For this review, use the dimensioned drawing (mm, ordinates from the lowest corner) and the shaded views. A direction names the side the tool comes from. Give positions to 0.01 mm unless a question says otherwise; leave off trailing zeros. Loops run counter-clockwise (first coordinate to the right, second up) from the corner with the lowest first, then second, coordinate; pieces in that order, holes last. Notation, with made-up numbers: M -16,-29 L 34,-29 A26 ccw 34,5 Z; hole C 65,-13.75 d1. An arc over 180 degrees is marked long. Use a Markdown table: item, result. Add a question column.
(1) For probe 1 along Z at (x, y) = (39, 13); probe 2 along Y at (x, z) = (55.5, 9.5) (1 decimal); probe 3 along Z at (x, y) = (60, 71.5) (1 decimal), list the stretches that pass through material, from the lowest coordinate up.
(2) Add section A-A, the plane z = 27. Give the boundary of the cut face in (x, y).
(3) For the marked faces 1 and 2, list the 3-axis set-ups (+Z, -Z, +X, -X, +Y, -Y) from which the entire face can be reached by the end or side of a thin tool; tool diameter is ignored.
(4) Insertion check: pin 1 Ø10 at (y, z) = (51, 18.5) entering from -X (1 decimal); pin 2 Ø10 at (y, z) = (25, 19) entering from -X (1 decimal); pin 3 Ø6 at (y, z) = (44, 33) entering from -X. Each pin has a flat end and moves straight along its axis. Give the tip position at first contact, or say it passes through.
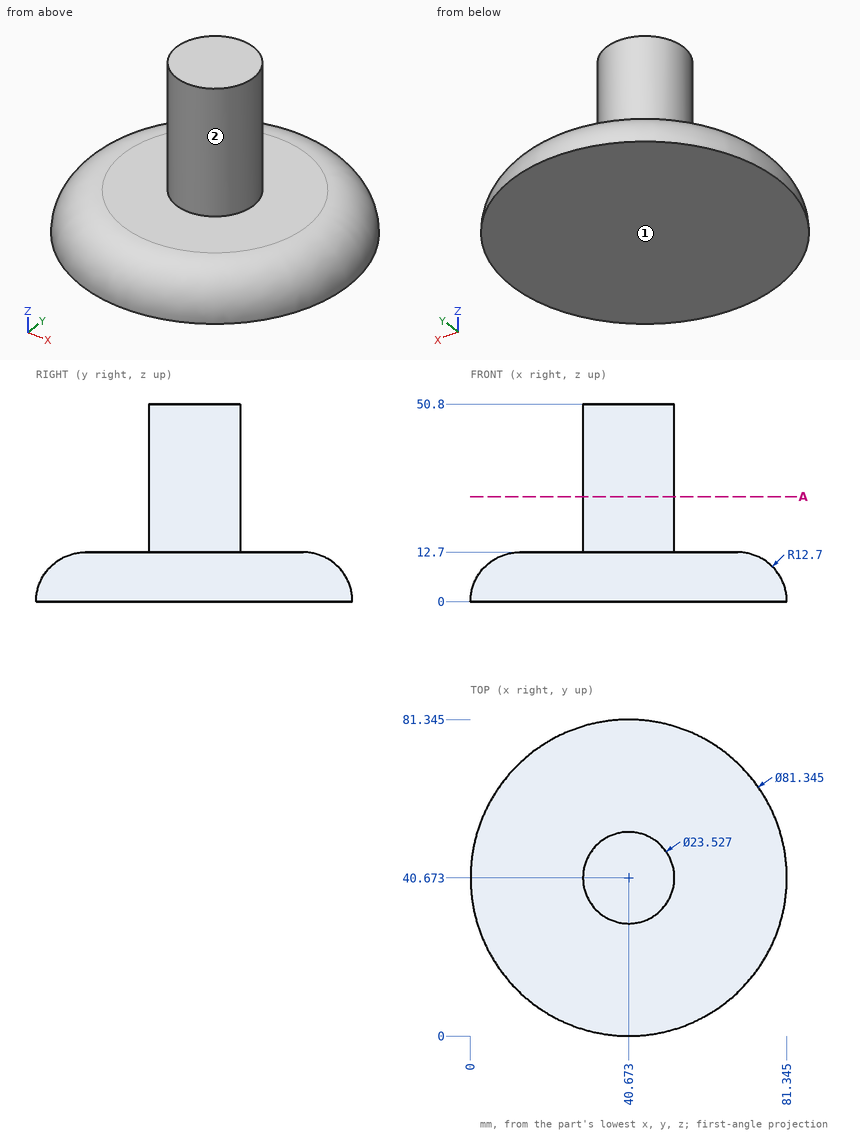
Established:
| question | item | result |
|---|---|---|
| 1 | probe 1 | 0 to 12.7 |
| 1 | probe 2 | 7.4 to 73.9 |
| 1 | probe 3 | 0 to 9.5 |
| 2 | outline | C 40.67,40.67 d23.53 |
| 3 | face 1 | -Z, +X, -X, +Y, -Y |
| 3 | face 2 | +Z |
| 4 | pin 1 | x = 30.2 |
| 4 | pin 2 | x = 35.7 |
| 4 | pin 3 | x = 28.91 |
